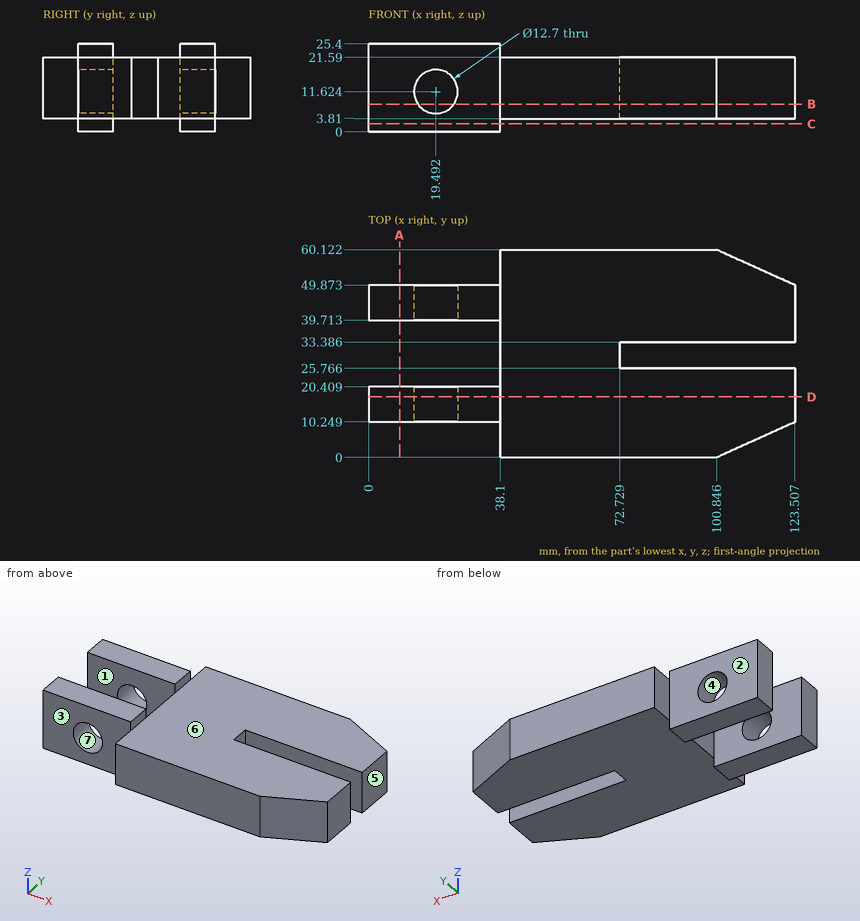
Study the drawing (mm; zero at the part's minimum x, y, z) and answer. A direction names the side the tool comes from. Round coordinates to 2 decimals unless told otherwise and drop trailing zeros. Order: outer loops, then holes, each group sorted by start corner. A loop starts at its lowest first (then second) coordinate and runs counter-clockwise, first axis right, second up. Notation, with made-up numbers: M 70,13 L 100,13 A27 cw 100,45 Z; hole C 63,67 d11. An arc over 180 degrees is marked long. One line per item, written item: value.
Q1. Find section D-D on y = 17.5. Write down the section's boundary in (x, z).
Derived:
outline: M 0,0 L 38.1,0 L 38.1,3.81 L 123.51,3.81 L 123.51,21.59 L 38.1,21.59 L 38.1,25.4 L 0,25.4 Z; hole C 19.49,11.62 d12.7
Q2. Determine the mould class of the marked faces 4, 5, 6 and 7 for opening direction Z: released by +Z, released by -Z, zero draft, split by the parting line, or undercut.
Derived:
face 4: undercut
face 5: zero draft
face 6: released by +Z
face 7: undercut
Q3. Flat-ended cylindrical pins translate along their axes: pin 1 (5 mm diameter, centred on y = 55.5, z = 11, fed in from -X); pin 2 (12 mm diameter, centred on x = 67.5, y = 46, fed in from +Z); pin 3 (7.5 mm diameter, centred on x = 27, z = 8.5, fed in from -Y). Find the tip coordinate at first contact, or state that the pin passes through.
Derived:
pin 1: x = 38.1
pin 2: z = 21.59
pin 3: y = 10.25
Q4. Find section A-A on x = 9. Write down the section's boundary in (y, z).
Derived:
outline: M 10.25,0 L 20.41,0 L 20.41,25.4 L 10.25,25.4 Z; M 39.71,0 L 49.87,0 L 49.87,25.4 L 39.71,25.4 Z
Q5. For the marked faces 1, 2 and 3, determine the directions among +Z, -Z, +X, -X, +Y, -Y from which every point of the face is accessible in a straight line to the end or side of a thin tool.
Derived:
face 1: +Z, -Z, -X
face 2: +Z, -Z, -X, +Y
face 3: +Z, -Z, -X, -Y
Q6. Find section B-B on z = 8. Give the number of separate pieces and of enclosed holes in the cut face, then the cut area to 3 significant figures.
Derived:
separate pieces: 3
enclosed holes: 0
area: 5,080 mm²
Q7. Straight lines are drawn through the part: line 1 (Y direction, x = 79.5, z = 10) (1 decimal); line 2 (Y direction, x = 14, z = 6.25); line 3 (Z direction, x = 49.5, y = 3). For each, find the intervals that lie inside material, in ascending order.
Derived:
line 1: 0 to 25.8, 33.4 to 60.1
line 2: 10.25 to 20.41, 39.71 to 49.87
line 3: 3.81 to 21.59
Q8. Find section C-C on z = 2.25. Write down the section's boundary in (x, y), then the cut area to 3 significant figures.
Derived:
outline: M 0,10.25 L 38.1,10.25 L 38.1,20.41 L 0,20.41 Z; M 0,39.71 L 38.1,39.71 L 38.1,49.87 L 0,49.87 Z
area: 774 mm²
